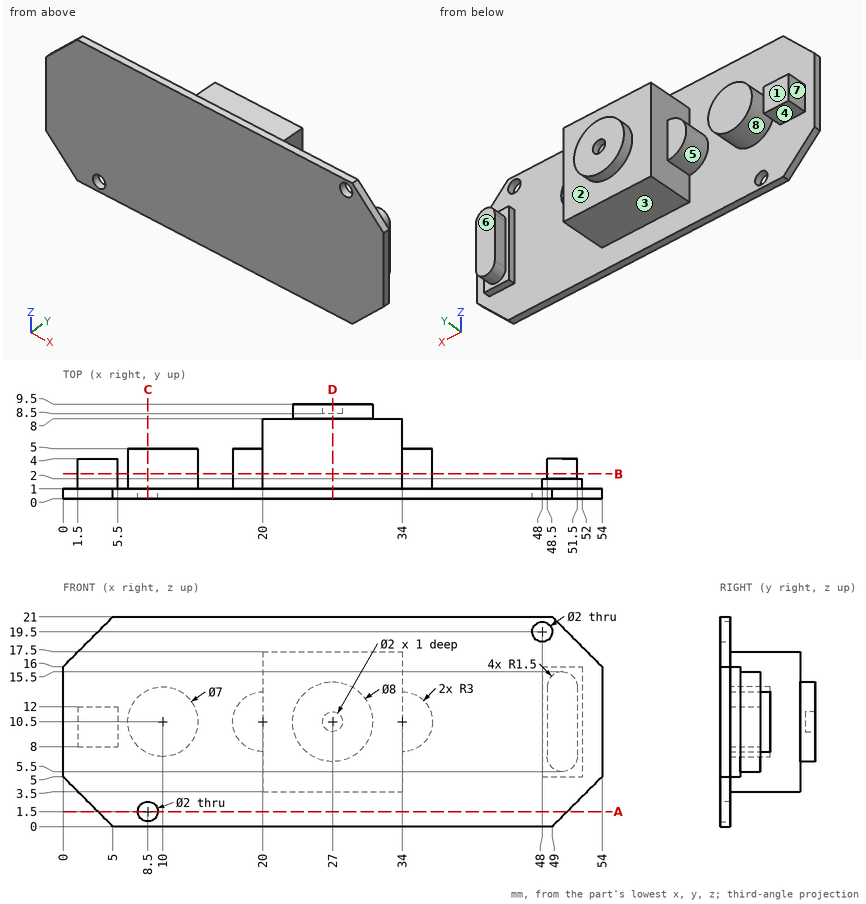
Print and shaded views of the part. All mm, measured from the part's lowest x, y and z. A direction names the side the tool comes from. Round coordinates to 2 decimals unless told otherwise and drop trailing zeros. Write each loop counter-clockwise with the first axis right and the second up, starting at its lowest first coordinate (ties: lowest second). Pieces come first, ordered by that corner, then holes. Notation, with made-up numbers: (-30, 56.25) - (18, 56.25) arc R26 cw to (18, 92.25) - close; hole circle Ø9 at (15, 40). An arc over 180 degrees is marked (long way). Use CSV: the item, a comma, the result in double quotes. Start each with the question number.
Item 1: Drill centre lines: L1, parallel to X at y = 3.5, z = 11.5; L2, parallel to X at y = 2.25, z = 9.75 (1 decimal); L3, parallel to Z at x = 48, y = 0.3. Where is each one in solid material? Low to high. Write a range as [from, to].
Item 2: Two-plate mould, pull along X, no slides. Class the marked faces 5, 6, 7 and 8: released by +X, released by -X, zero draft, split by the parting line, or undercut.
Item 3: Pin check, flat tips, straight feed: P1, Ø10, axis at x = 21.5, z = 12, coming from the -Y side; P2, Ø3, axis at x = 50, z = 8.5, coming from the +Y side; P3, Ø3.5, axis at y = 5.5, z = 10, coming from the -X side; P4, Ø12, axis at x = 12.5, z = 4.5, coming from the +Y side. Stop position of each tip, or through.
Item 4: Tool access for the marked faces 1, 2, 3 and 4: list every direction of +Z, -Z, +X, -X, +Y, -Y with a clear straight run to the whole face (end or side of a thin tool).
Item 5: Band-saw the part on A-A (z = 1.5). Write the cut outline in (x, y).
Item 6: Band-saw the part on B-B (y = 2.5). State how many separate pieces and enclosed holes the cut face has, and give its area (3 significant figures).
Item 7: Band-saw the part on C-C (x = 8.5). Write the cut outline in (y, z), and give its area (3 significant figures).
Item 8: Band-saw the part on D-D (x = 27). Write the cut outline in (y, z).
Checked values:
1,L1,"x = [1.5, 5.5], [6.65, 13.35], [17.17, 36.83], [48.5, 51.5]"
1,L2,"x = [1.5, 5.5], [6.6, 13.4], [17.1, 36.9], [48.5, 51.5]"
1,L3,"z = [0, 18.5], [20.5, 21]"
2,face 5,"undercut"
2,face 6,"zero draft"
2,face 7,"released by -X"
2,face 8,"undercut"
3,P1,"stops at y = 0"
3,P2,"stops at y = 4"
3,P3,"stops at x = 1.5"
3,P4,"stops at y = 5"
4,face 1,"+Z, -Z, -X, +Y"
4,face 2,"+Y"
4,face 3,"-Z, +X, -X, +Y"
4,face 4,"-Z, -X, +Y"
5,outline,"(3.5, 0) - (7.5, 0) - (7.5, 1) - (3.5, 1) - close; (9.5, 0) - (50.5, 0) - (50.5, 1) - (9.5, 1) - close"
6,separate pieces,"4"
6,enclosed holes,"0"
6,area,"307 mm²"
7,outline,"(0, 0) - (1, 0) - (1, 0.5) - (0, 0.5) - close; (0, 2.5) - (1, 2.5) - (1, 7.34) - (5, 7.34) - (5, 13.66) - (1, 13.66) - (1, 21) - (0, 21) - close"
7,area,"44.3 mm²"
8,outline,"(0, 0) - (1, 0) - (1, 3.5) - (8, 3.5) - (8, 6.5) - (9.5, 6.5) - (9.5, 9.5) - (8.5, 9.5) - (8.5, 11.5) - (9.5, 11.5) - (9.5, 14.5) - (8, 14.5) - (8, 17.5) - (1, 17.5) - (1, 21) - (0, 21) - close"
